Part model, mm, in its own coordinate system. Face numbers are marked on the shaded views. A direction names the side the tool comes from. Give positions to 0.01 mm unless a question says otherwise; leave off trailing zeros. Write each loop counter-clockwise with the first axis right and the second up, starting at its lowest first coordinate (ties: lowest second). Pieces come first, ordered by that corner, then holes. Notation, with made-up numbers: M 0,27.5 L 54,27.5 A13 ccw 54,44.5 Z; hole C 17,44.25 d8. An arc over 180 degrees is marked long. Use a Markdown table: item, result.
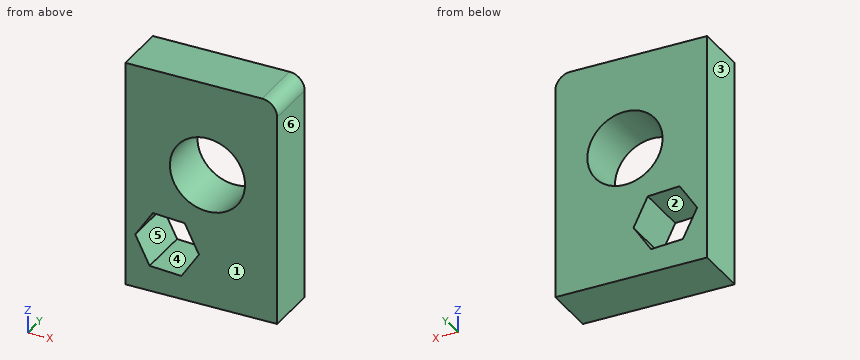
```python
from build123d import *

# Parameters (mm, degrees)
F0_W     = 100
F0_H     = 150
F1_DEPTH = 35
F2_R     = 24.758071
F3_DEPTH = 93
F4_R     = 10


with BuildPart() as f1:
    # F0 (on Front) → F1 (new body)
    with BuildSketch(Plane.XZ):
        with Locations((1.924342, 24.967596)):
            Rectangle(F0_W, F0_H)
    extrude(amount=F1_DEPTH)

    # F2 (on face) → F3 (cut)
    with BuildSketch(Plane.XZ.offset(35)):
        with Locations((6.043291, 38.55627)):
            Circle(F2_R)
        Polygon((-11.134558, -34.447833), (0.429299, -16.902675), (-8.983325, 1.884497), (-29.959805, 3.126512), (-41.523662, -14.418645), (-32.111038, -33.205818), align=None)
    extrude(amount=-F3_DEPTH, mode=Mode.SUBTRACT)

    # F4
    f4_edges = [f1.edges().sort_by_distance(p)[0] for p in [
        (51.924342, -17.5, 99.967596),
    ]]
    fillet(f4_edges, radius=F4_R)


solid = f1.part
```
1. Drill centre lines: L1, parallel to Z at x = 5.5, y = -15.5; L2, parallel to Z at x = -8, y = -24; L3, parallel to X at y = -2, z = -24.5. Where is each one in solid material? Low to high.
Findings below:
| item | result |
|---|---|
| L1 | -50.03 to 13.8, 63.31 to 99.97 |
| L2 | -50.03 to -29.69, -0.08 to 18.17, 58.95 to 99.97 |
| L3 | -48.08 to -36.47, -4.58 to 51.92 |
2. Cut at C-C, the plane y = -13. Give the cut face in (x, z).
Findings below:
| item | result |
|---|---|
| outline | M -48.08,-50.03 L 51.92,-50.03 L 51.92,89.97 A10 ccw 41.92,99.97 L -48.08,99.97 Z; hole M -41.52,-14.42 L -32.11,-33.21 L -11.13,-34.45 L 0.43,-16.9 L -8.98,1.88 L -29.96,3.13 Z; hole C 6.04,38.56 d49.52 |
3. Two-plate mould, pull along X, no slides. Class the marked faces 1, 2, 3 and 4: released by +X, released by -X, zero draft, split by the parting line, or undercut.
Findings below:
| item | result |
|---|---|
| face 1 | zero draft |
| face 2 | undercut |
| face 3 | released by -X |
| face 4 | undercut |
4. Cut at D-D, the plane x = -15.5. Give the cut face in (y, z).
Findings below:
| item | result |
|---|---|
| outline | M -35,-50.03 L 0,-50.03 L 0,-34.19 L -35,-34.19 Z; M -35,2.27 L 0,2.27 L 0,26.36 L -35,26.36 Z; M -35,50.76 L 0,50.76 L 0,99.97 L -35,99.97 Z |
5. Tool access for the marked faces 5 and 6: list every direction of +Z, -Z, +X, -X, +Y, -Y with a clear straight run to the whole face (end or side of a thin tool).
Findings below:
| item | result |
|---|---|
| face 5 | +Y, -Y |
| face 6 | +Z, -Z, +X, +Y, -Y |
6. Cut at A-A, the plane z = 35. Give the cut face in (x, y), then the cut area to 3 significant figures.
Findings below:
| item | result |
|---|---|
| outline | M -48.08,-35 L -18.46,-35 L -18.46,0 L -48.08,0 Z; M 30.54,-35 L 51.92,-35 L 51.92,0 L 30.54,0 Z |
| area | 1,780 mm2 |
7. Cut at B-B, the plane x = 15.5. Give the cut face in (y, z).
Findings below:
| item | result |
|---|---|
| outline | M -35,-50.03 L 0,-50.03 L 0,15.68 L -35,15.68 Z; M -35,61.44 L 0,61.44 L 0,99.97 L -35,99.97 Z |
